from build123d import *

# Parameters (mm, degrees)
F0_W     = 550
F0_H     = 550
F1_DEPTH = 50
F2_W     = 52
F2_H     = 52
F3_DEPTH = 400
F4_W     = 58.6
F4_H     = 58.6
F5_DEPTH = 50


with BuildPart() as f1:
    # F0 (on Top) → F1 (new body)
    with BuildSketch(Plane.XY):
        Rectangle(F0_W, F0_H)
    extrude(amount=F1_DEPTH)

    # F2 (on face) → F3 (join)
    with BuildSketch(Plane(origin=(0, 0, 0), x_dir=(1, 0, 0), z_dir=(0, 0, -1))):
        with Locations((-248, 248)):
            Rectangle(F2_W, F2_H)
        with Locations((248, 248)):
            Rectangle(F2_W, F2_H)
        with Locations((248, -248)):
            Rectangle(F2_W, F2_H)
        with Locations((-248, -248)):
            Rectangle(F2_W, F2_H)
    extrude(amount=F3_DEPTH)

    # F4 (on face) → F5 (join)
    with BuildSketch(Plane(origin=(0, 0, -400), x_dir=(1, 0, 0), z_dir=(0, 0, -1))):
        with Locations((-248, -248)):
            Rectangle(F4_W, F4_H)
    extrude(amount=F5_DEPTH)


solid = f1.part
Work out the finished part from the listing and answer in its coordinate system (mm). A direction names the side the tool comes from. Give positions to 0.01 mm unless a question says otherwise; leave off trailing zeros. Write each loop counter-clockwise with the first axis right and the second up, starting at its lowest first coordinate (ties: lowest second). Pieces come first, ordered by that corner, then holes. Notation, with made-up numbers: M -13,76 L 31,76 A26 cw 31,95 Z; hole C 4.25,-1 d11. An arc over 180 degrees is marked long. Answer as CSV lines item,"result".
Q1. Find the intervals of material crossed by probe 1 along Y at (x, z) = (-239.5, -306); probe 2 along Z at (x, y) = (218, 130); probe 3 along X at (y, z) = (-19.5, 17), in increasing order. Write a range as [from, to].
A:
probe 1,"y = [-274, -222], [222, 274]"
probe 2,"z = [0, 50]"
probe 3,"x = [-275, 275]"
Q2. A tool of negligible diameter and unlimited length cuts with its end or side. For faces 5 (the flat face through (248, 274, -197)), 6 (the flat face through (-248, -248, -400)), 7 (the flat face through (-222, 248, -197)), 8 (the flat face through (-274, -248, -197)), from which of +Z, -Z, +X, -X, +Y, -Y can it reach the whole face along a straight path? Write none if from no direction.
A:
face 5,"-Z, +X, -X, +Y"
face 6,"-Z, +X, -X, -Y"
face 7,"+Y, -Y"
face 8,"-Z, -X, +Y, -Y"
Q3. A cutting plane is placed at C-C on y = 175.5. Write down the section's boundary in (x, z), plus the area to 3 significant figures.
A:
outline,"M -275,0 L 275,0 L 275,50 L -275,50 Z"
area,"27,500 mm²"
Q4. A cutting plane is placed at A-A on z = -317. Write down the section's boundary in (x, y), plus the area to 3 significant figures.
A:
outline,"M -274,-274 L -222,-274 L -222,-222 L -274,-222 Z; M -274,222 L -222,222 L -222,274 L -274,274 Z; M 222,-274 L 274,-274 L 274,-222 L 222,-222 Z; M 222,222 L 274,222 L 274,274 L 222,274 Z"
area,"10,800 mm²"
Q5. Given P1, Ø12, axis at x = 146, y = -187.5, coming from the -Z side; P2, Ø15, axis at y = -32, z = 25, coming from the -X side; P3, Ø15.5, axis at x = 247.5, y = -247, coming from the -Z side, each flat-ended and moving along its own axis, determine where each tip first touches the part or whether it passes through.
A:
P1,"stops at z = 0"
P2,"stops at x = -275"
P3,"stops at z = -400"
Q6. The mould has two halves that part along Y. Classify faces 1 (the flat face through (-248, 222, -197)), 2 (the flat face through (222, 248, -197)), 3 (the flat face through (-248, -222, -197)), 4 (the flat face through (-4, 275, 25)): +Y half, -Y half, draft (parallel to the pull), parting line (faces both ways), or undercut.
A:
face 1,"undercut"
face 2,"draft"
face 3,"undercut"
face 4,"+Y half"
Q7. A cutting plane is placed at B-B on x = -232.5. Write down the section's boundary in (y, z), plus the area to 3 significant figures.
A:
outline,"M -275,0 L -274,0 L -274,-400 L -222,-400 L -222,0 L 222,0 L 222,-400 L 218.7,-400 L 218.7,-450 L 277.3,-450 L 277.3,-400 L 274,-400 L 274,0 L 275,0 L 275,50 L -275,50 Z"
area,"72,000 mm²"
